Check sheet for the drawn part. Datum: minimum x, y, z corner. Units: mm. Coordinates: 2 decimals unless noted, no trailing zeros. Write each loop counter-clockwise with the first axis right and the second up, starting at its lowest first coordinate (ties: lowest second). Pieces come first, ordered by that corner, then holes. Notation, with made-up numbers: (26, 83.5) -> (56, 83.5) arc R7 ccw to (56, 91.5) -> close; hole circle Ø3 at (31.25, -38.75). An arc over 180 degrees is marked (long way). One line per question, with ' | ' between items.
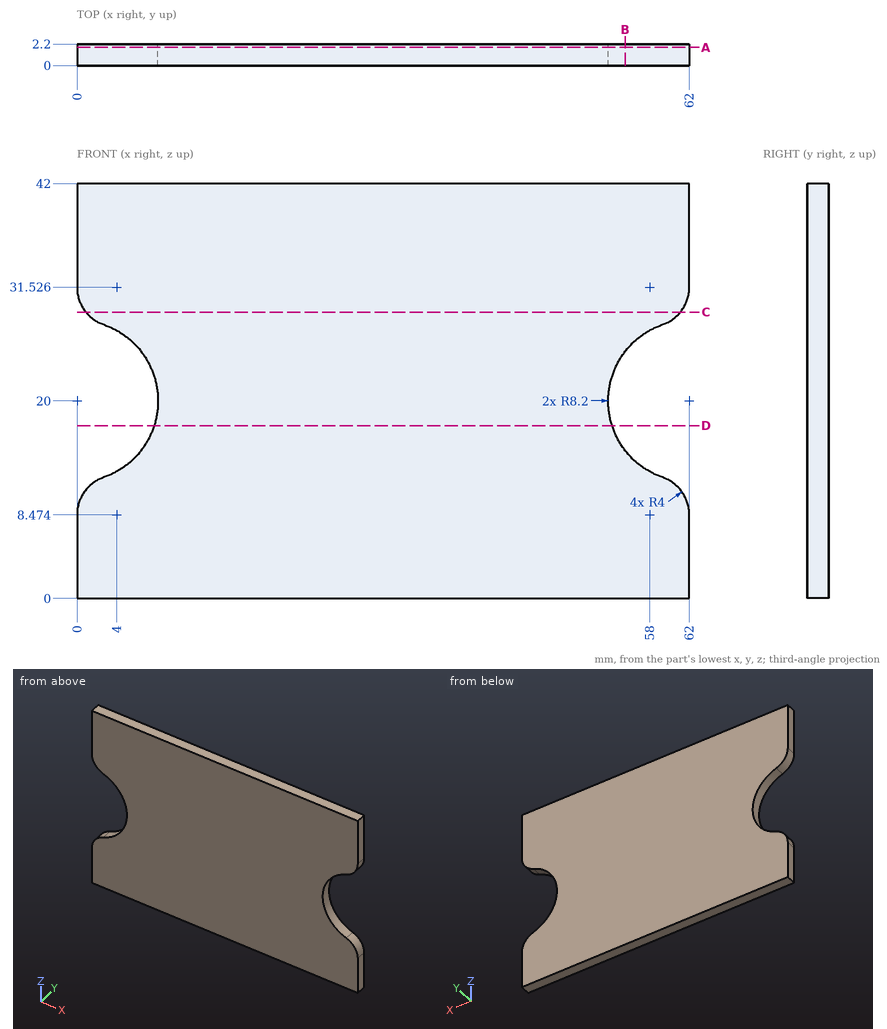
1. Cross-section at D-D on z = 17.5. Record the boundary of the cut face in (x, y).
Worked answers:
outline: (7.81, 0) -> (54.19, 0) -> (54.19, 2.2) -> (7.81, 2.2) -> close
2. Cross-section at C-C on z = 29. Record the boundary of the cut face in (x, y).
Worked answers:
outline: (0.9, 0) -> (61.1, 0) -> (61.1, 2.2) -> (0.9, 2.2) -> close
3. Material ranges on line 1 (Z direction, x = 3, y = 0.25); line 2 (Z direction, x = 58.5, y = 0.85) (1 decimal); line 3 (X direction, y = 1.5, z = 17), recorded low to high. Write a range as from..to.
Worked answers:
line 1: 0..12.37, 27.63..42 | line 2: 0..12.6, 27.4..42 | line 3: 7.63..54.37
4. Cross-section at B-B on x = 55.5. Record the boundary of the cut face in (y, z).
Worked answers:
outline: (0, 0) -> (2.2, 0) -> (2.2, 15) -> (0, 15) -> close; (0, 25) -> (2.2, 25) -> (2.2, 42) -> (0, 42) -> close
5. Go/stop test with a flat-tipped pin: P1, Ø2, axis at x = 33.5, z = 36, coming from the -Y side. Record where the tip stops, or that it passes through.
Worked answers:
P1: y = 0
6. Cross-section at A-A on y = 1.85. Record the boundary of the cut face in (x, z) (1 decimal).
Worked answers:
outline: (0, 0) -> (62, 0) -> (62, 8.5) arc R4 ccw to (59.3, 12.3) arc R8.2 cw to (59.3, 27.7) arc R4 ccw to (62, 31.5) -> (62, 42) -> (0, 42) -> (0, 31.5) arc R4 ccw to (2.7, 27.7) arc R8.2 cw to (2.7, 12.3) arc R4 ccw to (0, 8.5) -> close
